Geometry: final body of the model. Coordinates: model frame, mm. Face numbers are marked on the shaded views. A direction names the side the tool comes from. Give positions to 0.01 mm unless a question says otherwise; leave off trailing zeros. Write each loop counter-clockwise with the first axis right and the second up, starting at its lowest first coordinate (ties: lowest second). Pieces come first, ordered by that corner, then holes. Notation, with made-up numbers: (59, 62.25) -> (69, 62.25) arc R19 cw to (69, 79.25) -> close; hole circle Ø11 at (1.25, 15.25). An arc over 180 degrees is marked (long way). Answer as a JSON object with one key per item and string values.
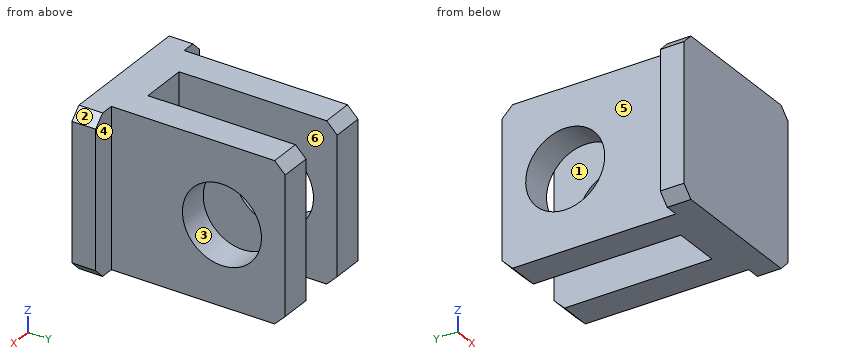
from build123d import *

# Parameters (mm, degrees)
SKETCH_1_W          = 30
SKETCH_1_H          = 37.5
EXTRUDE_1_DEPTH     = 15
CHAMFER_1_SIZE      = 2
CUT_EXTRUDE_1_REACH = 32
SKETCH_2_W          = 4.5
SKETCH_2_H          = 33
SKETCH_2_W_2        = 9
SKETCH_2_H_2        = 30
SKETCH_3_R          = 7.5
CUT_EXTRUDE_2_DEPTH = 10.5
CHAMFER_2_SIZE      = 2


with BuildPart() as part:
    # 스케치1 → 보스-돌출1 (new body, symmetric)
    with BuildSketch(Plane(origin=(0, 0, 0), x_dir=(0, 0, -1), z_dir=(1, 0, 0))):
        with Locations((15, 18.75)):
            Rectangle(SKETCH_1_W, SKETCH_1_H)
    extrude(amount=EXTRUDE_1_DEPTH, both=True)

    # 모따기1
    chamfer_1_edges = [part.edges().sort_by_distance(p)[0] for p in [
        (0, 37.5, 0),
        (0, 37.5, -30),
    ]]
    chamfer(chamfer_1_edges, length=CHAMFER_1_SIZE)

    # 스케치2 → 컷-돌출1 (cut, up to next)
    with BuildSketch(Plane.XY, mode=Mode.PRIVATE) as cut_extrude_1_sk1:
        with Locations((-12.75, 21)):
            Rectangle(SKETCH_2_W, SKETCH_2_H)
    cut_extrude_1_tool1 = extrude(cut_extrude_1_sk1.sketch, amount=-CUT_EXTRUDE_1_REACH, mode=Mode.PRIVATE) & part.part
    add(cut_extrude_1_tool1.solids().sort_by_distance((-12.75, 21, 0))[0], mode=Mode.SUBTRACT)
    # 스케치2 → 컷-돌출1 (cut, up to next)
    with BuildSketch(Plane.XY, mode=Mode.PRIVATE) as cut_extrude_1_sk2:
        with Locations((12.75, 21)):
            Rectangle(SKETCH_2_W, SKETCH_2_H)
    cut_extrude_1_tool2 = extrude(cut_extrude_1_sk2.sketch, amount=-CUT_EXTRUDE_1_REACH, mode=Mode.PRIVATE) & part.part
    add(cut_extrude_1_tool2.solids().sort_by_distance((12.75, 21, 0))[0], mode=Mode.SUBTRACT)
    # 스케치2 → 컷-돌출1 (cut, up to next)
    with BuildSketch(Plane.XY, mode=Mode.PRIVATE) as cut_extrude_1_sk3:
        with Locations((0, 22.5)):
            Rectangle(SKETCH_2_W_2, SKETCH_2_H_2)
    cut_extrude_1_tool3 = extrude(cut_extrude_1_sk3.sketch, amount=-CUT_EXTRUDE_1_REACH, mode=Mode.PRIVATE) & part.part
    add(cut_extrude_1_tool3.solids().sort_by_distance((0, 22.5, 0))[0], mode=Mode.SUBTRACT)

    # 스케치3 → 컷-돌출2 (cut, symmetric)
    with BuildSketch(Plane(origin=(0, 0, 0), x_dir=(0, 0, -1), z_dir=(1, 0, 0))):
        with Locations((15, 25.5)):
            Circle(SKETCH_3_R)
    extrude(amount=CUT_EXTRUDE_2_DEPTH, both=True, mode=Mode.SUBTRACT)

    # 모따기2
    chamfer_2_edges = [part.edges().sort_by_distance(p)[0] for p in [
        (15, 2.25, -30),
        (-15, 2.25, 0),
        (15, 2.25, 0),
        (-15, 2.25, -30),
    ]]
    chamfer(chamfer_2_edges, length=CHAMFER_2_SIZE)


solid = part.part
Q1. Cut plane D-D (x = 5.75). Return the cut outline in (y, z), and give its area (3 significant figures).
Values:
{"outline": "(0, -30) -> (35.5, -30) -> (37.5, -28) -> (37.5, -2) -> (35.5, 0) -> (0, 0) -> close; hole circle Ø15 at (25.5, -15)", "area": "944 mm²"}
Q2. Cut plane A-A (z = -15). Return the cut outline in (x, y).
Values:
{"outline": "(-15, 0) -> (15, 0) -> (15, 4.5) -> (10.5, 4.5) -> (10.5, 18) -> (4.5, 18) -> (4.5, 7.5) -> (-4.5, 7.5) -> (-4.5, 18) -> (-10.5, 18) -> (-10.5, 4.5) -> (-15, 4.5) -> close; (-10.5, 33) -> (-4.5, 33) -> (-4.5, 37.5) -> (-10.5, 37.5) -> close; (4.5, 33) -> (10.5, 33) -> (10.5, 37.5) -> (4.5, 37.5) -> close"}
Q3. Cut plane B-B (y = 25.5). Return the cut outline in (x, z), and give its area (3 significant figures).
Values:
{"outline": "(-10.5, -30) -> (-4.5, -30) -> (-4.5, -22.5) -> (-10.5, -22.5) -> close; (-10.5, -7.5) -> (-4.5, -7.5) -> (-4.5, 0) -> (-10.5, 0) -> close; (4.5, -30) -> (10.5, -30) -> (10.5, -22.5) -> (4.5, -22.5) -> close; (4.5, -7.5) -> (10.5, -7.5) -> (10.5, 0) -> (4.5, 0) -> close", "area": "180 mm²"}
Q4. First-contact query: P1, Ø13.5, axis at y = 25.5, z = -15, coming from the -X side; P2, Ø15, axis at y = 20.5, z = -8.5, coming from the +X side; P3, Ø15, axis at y = 24, z = -15.5, coming from the -X side; P4, Ø5, axis at x = 14, z = -21.5, coming from the +Y side. Flat tips, straight axial feed; report the tip coordinate or a pass-through.
Values:
{"P1": "through", "P2": "x = 10.5", "P3": "x = -10.5", "P4": "y = 4.5"}
Q5. Set-up query: the marked faces 4, 5 and 6. Return all of +Z, -Z, +X, -X, +Y, -Y with unobstructed straight access to the full face (end or side cutting, diameter ignored); none if empty.
Values:
{"face 4": "+Z, -Z, +X, +Y", "face 5": "+Z, -Z, -X, +Y", "face 6": "+Z, -Z, +Y"}
Q6. Cut plane C-C (y = 10). Return the cut outline in (x, z), and give its area (3 significant figures).
Values:
{"outline": "(-10.5, -30) -> (-4.5, -30) -> (-4.5, 0) -> (-10.5, 0) -> close; (4.5, -30) -> (10.5, -30) -> (10.5, 0) -> (4.5, 0) -> close", "area": "360 mm²"}
Q7. Material intervals for L1, parallel to X at y = 14, z = -15; L2, parallel to Y at x = 9.25, z = -14.75; L3, parallel to Y at x = -2, z = -15.75, sorted ascending. Write a range as from..to.
Values:
{"L1": "-10.5..-4.5, 4.5..10.5", "L2": "0..18, 33..37.5", "L3": "0..7.5"}
Q8. Mould query, pull axis Z, two halves, no side actions, for the marked faces 1, 2 and 3. Classes: pulls with the +Z half, pulls with the -Z half, needs draft (parallel to the pull), parting line crosses it, or undercut.
Values:
{"face 1": "needs draft", "face 2": "pulls with the +Z half", "face 3": "undercut"}
